```python
from build123d import *

# Parameters (mm, degrees)
SKETCH1_W           = 144
SKETCH1_H           = 35
BOSS_EXTRUDE1_DEPTH = 7
BOSS_EXTRUDE2_DEPTH = 7
SKETCH8_W           = 58
SKETCH8_H           = 32.108669786
CUT_EXTRUDE5_DEPTH  = 84.900238379
FILLET1_R           = 7
CUT_EXTRUDE3_DEPTH  = 84.900238379
CUT_EXTRUDE4_DEPTH  = 2.5
CHAMFER2_SIZE       = 2.5
CHAMFER3_SIZE       = 1


with BuildPart() as part:
    # Sketch1 → Boss-Extrude1 (new body)
    with BuildSketch(Plane(origin=(0, 0, 0), x_dir=(1, 0, 0), z_dir=(0, 1, 0))):
        Rectangle(SKETCH1_W, SKETCH1_H)
        with BuildLine():
            Line((-55.125, 3.06794739), (-57.5, -2.108669786))
            Line((-57.5, -2.108669786), (-57.5, -9.608669786))
            Line((-57.5, -9.608669786), (-66.5, -9.608669786))
            Line((-66.5, -9.608669786), (-66.5, -14.608669786))
            Line((-66.5, -14.608669786), (-35.5, -14.608669786))
            Line((-35.5, -14.608669786), (-35.5, -9.608669786))
            Line((-35.5, -9.608669786), (-44.5, -9.608669786))
            Line((-44.5, -9.608669786), (-44.5, -2.108669786))
            Line((-44.5, -2.108669786), (-46.875, 3.06794739))
            ThreePointArc((-46.875, 3.06794739), (-51, 14.591330214), (-55.125, 3.06794739))
        make_face(mode=Mode.SUBTRACT)
        with BuildLine():
            Line((46.875, 3.06794739), (44.5, -2.108669786))
            Line((44.5, -2.108669786), (44.5, -9.608669786))
            Line((44.5, -9.608669786), (35.5, -9.608669786))
            Line((35.5, -9.608669786), (35.5, -14.608669786))
            Line((35.5, -14.608669786), (66.5, -14.608669786))
            Line((66.5, -14.608669786), (66.5, -9.608669786))
            Line((66.5, -9.608669786), (57.5, -9.608669786))
            Line((57.5, -9.608669786), (57.5, -2.108669786))
            Line((57.5, -2.108669786), (55.125, 3.06794739))
            ThreePointArc((55.125, 3.06794739), (51, 14.591330214), (46.875, 3.06794739))
        make_face(mode=Mode.SUBTRACT)
    extrude(amount=BOSS_EXTRUDE1_DEPTH)

    # Sketch6 → Boss-Extrude2 (add)
    with BuildSketch(Plane(origin=(0, 7, 0), x_dir=(1, 0, 0), z_dir=(0, 1, 0))):
        Polygon((72, -17.5), (39.577085299, -42.5), (-39.577085299, -42.5), (-72, -17.5), align=None)
    extrude(amount=-BOSS_EXTRUDE2_DEPTH)

    # Sketch8 → Cut-Extrude5 (cut, through all)
    with BuildSketch(Plane(origin=(0, 7, 0), x_dir=(1, 0, 0), z_dir=(0, 1, 0))):
        with Locations((0, 1.445665107)):
            Rectangle(SKETCH8_W, SKETCH8_H)
    extrude(amount=-CUT_EXTRUDE5_DEPTH, mode=Mode.SUBTRACT)

    # Fillet1
    fillet1_edges = [part.edges().sort_by_distance(p)[0] for p in [
        (29, 3.5, -17.5),
        (29, 3.5, 14.608669786),
        (-72, 3.5, -17.5),
        (72, 3.5, -17.5),
        (39.577085299, 3.5, 42.5),
        (-39.577085299, 3.5, 42.5),
        (72, 3.5, 17.5),
        (-72, 3.5, 17.5),
        (-29, 3.5, 14.608669786),
        (-29, 3.5, -17.5),
    ]]
    fillet(fillet1_edges, radius=FILLET1_R)

    # Sketch4 → Cut-Extrude3 (cut, through all)
    with BuildSketch(Plane(origin=(0, 7, 0), x_dir=(1, 0, 0), z_dir=(0, 1, 0))):
        with BuildLine():
            Line((-22.5, -26.804334893), (22.5, -26.804334893))
            ThreePointArc((22.5, -26.804334893), (24.25, -28.554334893), (22.5, -30.304334893))
            Line((22.5, -30.304334893), (-22.5, -30.304334893))
            ThreePointArc((-22.5, -30.304334893), (-24.25, -28.554334893), (-22.5, -26.804334893))
        make_face()
    extrude(amount=-CUT_EXTRUDE3_DEPTH, mode=Mode.SUBTRACT)

    # Sketch5 → Cut-Extrude4 (cut)
    with BuildSketch(Plane(origin=(0, 7, 0), x_dir=(1, 0, 0), z_dir=(0, 1, 0))):
        Polygon((-28.837742903, 35.825509873), (-28.837742903, -18.333082707), (-81.160450989, -18.333082707), (-81.160450989, -59.181512703), (81.160450989, -59.181512703), (81.160450989, -18.333082707), (28.837742903, -18.333082707), (28.837742903, 35.825509873), align=None)
    extrude(amount=-CUT_EXTRUDE4_DEPTH, mode=Mode.SUBTRACT)

    # Chamfer2
    chamfer2_edges = [part.edges().sort_by_distance(p)[0] for p in [
        (28.837742903, 4.5, 13.720087831),
        (49.690387643, 4.5, 18.333082707),
        (-28.837742903, 4.5, 13.720087831),
        (-49.690387643, 4.5, 18.333082707),
    ]]
    chamfer(chamfer2_edges, length=CHAMFER2_SIZE - 0.0001)  # a hair under: the kernel refuses the full size

    # Chamfer3
    chamfer3_edges = [part.edges().sort_by_distance(p)[0] for p in [
        (-51, 0, -14.591330214),
        (-56.3125, 0, -0.479638802),
        (-57.5, 0, 5.858669786),
        (-62, 0, 9.608669786),
        (-66.5, 0, 12.108669786),
        (-51, 0, 14.608669786),
        (-35.5, 0, 12.108669786),
        (-40, 0, 9.608669786),
        (-44.5, 0, 5.858669786),
        (-45.6875, 0, -0.479638802),
        (51, 0, -14.591330214),
        (45.6875, 0, -0.479638802),
        (44.5, 0, 5.858669786),
        (40, 0, 9.608669786),
        (35.5, 0, 12.108669786),
        (51, 0, 14.608669786),
        (66.5, 0, 12.108669786),
        (62, 0, 9.608669786),
        (57.5, 0, 5.858669786),
        (56.3125, 0, -0.479638802),
    ]]
    chamfer(chamfer3_edges, length=CHAMFER3_SIZE)


solid = part.part
```
The listing builds one solid part. Answer for the finished solid, in the listing's coordinates (mm). A direction names the side the tool comes from. Coordinates: 2 decimals unless noted, no trailing zeros. Loops run counter-clockwise (first coordinate to the right, second up) from the corner with the lowest first, then second, coordinate; pieces in that order, holes last. Notation, with made-up numbers: M -25,62.25 L -20,62.25 A24 ccw -20,73.25 Z; hole C 86,-14 d7. An arc over 180 degrees is marked long. Answer as a JSON object with one key per item and string values. Group by question number.
Item 1: Section B-B (y = 2.5) is taken. Give the number of separate pieces and of enclosed holes in the cut face, and give its area (3 significant figures).
Item 2: Consider L1, parallel to X at y = 3.75, z = 4.5; L2, parallel to X at y = 6.75, z = -5; L3, parallel to Z at x = -1.5, y = 2. Determine where each line is inside the solid, lowest interval first.
Item 3: Each of these flat-tipped pins is pushed along its axis until it touches: P1, Ø9, axis at x = -10.5, z = 31, coming from the +Y side; P2, Ø1.8, axis at x = -60, y = 3.5, coming from the +Z side; P3, Ø1.3, axis at x = 6.5, y = 3, coming from the -Z side. Where does it stop, or does it pass through?
Item 4: Section D-D (z = 23.5) is taken. Write down the section's boundary in (x, y), and give its area (3 significant figures).
Item 5: Which of the six approach directions +Z, -Z, +X, -X, +Y, -Y give full straight-line access (tool end or side, diameter ignored) to faces 4 (the face through (-66.5, 4, 12)), 5 (the face through (1, 2, 42.5)), 6 (the face through (56.82, 0.51, -0.55)), 7 (the face through (29, 4, -1))?
Item 6: Section A-A (x = -5.5) is taken. Write down the section's boundary in (y, z), and give its area (3 significant figures).
Item 7: Determine the mould class of faces 1 (the face through (50, 3, -17.5)), 2 (the face through (0, 2, 26.804)), 3 (the face through (39.48, 2.219, 42.115)) for opening direction X: +X half, -X half, draft (parallel to the pull), parting line (faces both ways), or undercut.
Solved:
{
 "1": {"separate pieces": "1", "enclosed holes": "3", "area": "4,910 mm2"},
 "2": {"L1": "x = -72 to -57.5, -44.5 to -29, 29 to 44.5, 57.5 to 72", "L2": "x = -72 to -56.72, -45.28 to -29, 29 to 45.28, 56.72 to 72", "L3": "z = 14.61 to 26.8, 30.3 to 42.5"},
 "3": {"P1": "stops at y = 4.5", "P2": "stops at z = 27.45", "P3": "stops at z = 14.61"},
 "4": {"outline": "M -64.22,0 L 64.22,0 L 64.22,4.5 L -64.22,4.5 Z", "area": "578 mm2"},
 "5": {"face 4": "+Y, -Y", "face 5": "+Z, +X, -X, +Y, -Y", "face 6": "-Y", "face 7": "-Z, +Y, -Y"},
 "6": {"outline": "M 0,14.61 L 4.5,14.61 L 4.5,26.8 L 0,26.8 Z; M 0,30.3 L 4.5,30.3 L 4.5,42.5 L 0,42.5 Z", "area": "110 mm2"},
 "7": {"face 1": "draft", "face 2": "undercut", "face 3": "+X half"}
}
